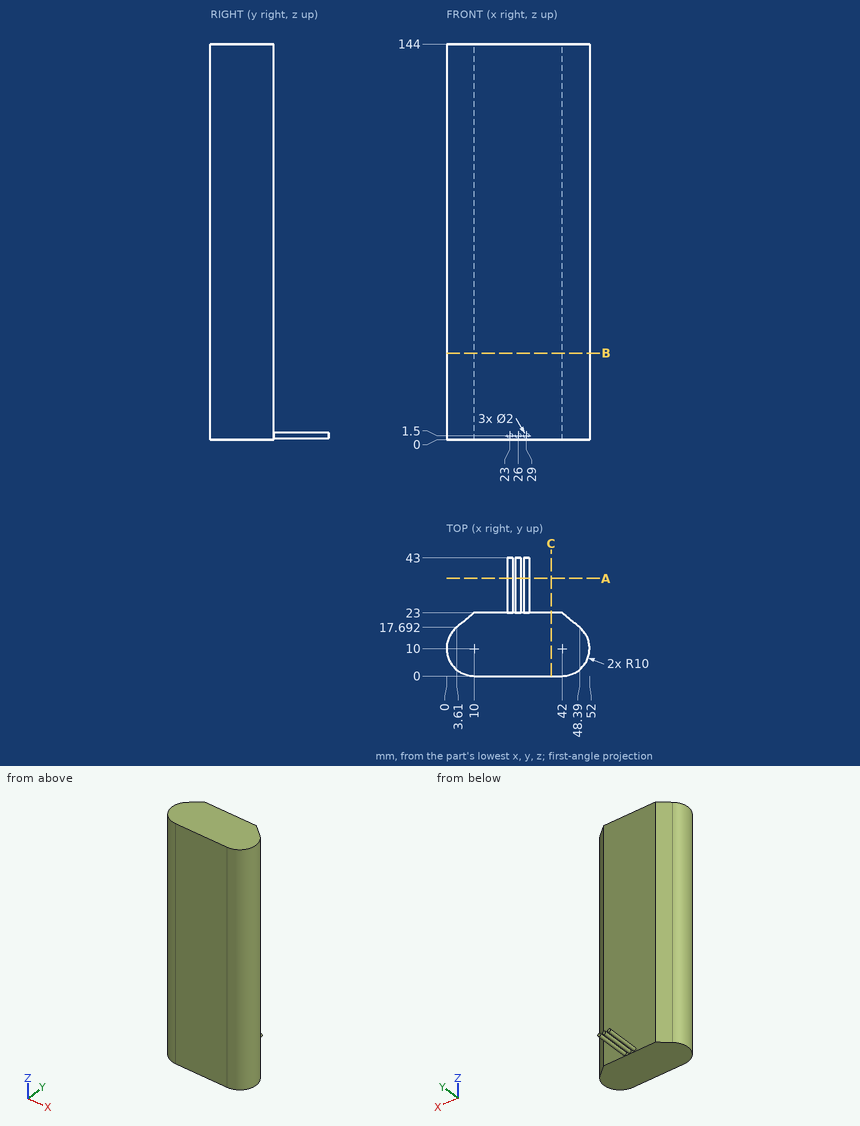
Job drawing, mm, ordinate dimensions from the low corner. One solid piece. Give positions to 0.01 mm unless a question says otherwise; leave off trailing zeros. Order: outer loops, then holes, each group sorted by start corner. A loop starts at its lowest first (then second) coordinate and runs counter-clockwise, first axis right, second up. Notation, with made-up numbers: (54, 38) - (91, 38) arc R33 ccw to (91, 76) - close; hole circle Ø3 at (-32, 85.5). An arc over 180 degrees is marked (long way). Answer in a Markdown table with one row per item.
1. Saw through at C-C, the plane x = 38. Give the cut face in (y, z).
Data:
| item | result |
|---|---|
| outline | (0, 0) - (23, 0) - (23, 144) - (0, 144) - close |
2. Saw through at A-A, the plane y = 35.5. Give the cut face in (x, z).
Data:
| item | result |
|---|---|
| outline | circle Ø2 at (23, 1.5); circle Ø2 at (26, 1.5); circle Ø2 at (29, 1.5) |
3. Probe probe 1 along Y at (x, z) = (38, 111); probe 2 along X at (y, z) = (14, 57.5) (1 decimal); probe 3 along X at (y, z) = (22.5, 60). List the from-to ranges inside material, lowest first. Write a range as [from, to].
Data:
| item | result |
|---|---|
| probe 1 | y = [0, 23] |
| probe 2 | x = [0.8, 51.2] |
| probe 3 | x = [9.4, 42.6] |
4. Saw through at B-B, the plane z = 31.5. Give the cut face in (x, y), plus the area to 3 significant figures.
Data:
| item | result |
|---|---|
| outline | (3.61, 17.69) arc R10 ccw to (10, 0) - (42, 0) arc R10 ccw to (48.39, 17.69) - (42, 23) - (10, 23) - close |
| area | 1,060 mm² |
5. Flat gauge pins, fed straight in: pin 1 (5 mm diameter, centred on x = 27.5, y = 32.5, fed in from -Z); pin 2 (4 mm diameter, centred on x = 25.5, z = 45.5, fed in from +Y); pin 3 (5 mm diameter, centred on y = 26, z = 97, fed in from +X). Where does each tip first touch, or does it go through?
Data:
| item | result |
|---|---|
| pin 1 | stops at z = 0.5 |
| pin 2 | stops at y = 23 |
| pin 3 | passes through |
